from build123d import *

# Parameters (mm, degrees)
SKETCH1_R           = 34.5
BOSS_EXTRUDE1_DEPTH = 3
SKETCH4_R           = 20
CUT_EXTRUDE2_DEPTH  = 49.88251221
SKETCH5_W           = 5
SKETCH5_H           = 5
CUT_EXTRUDE3_DEPTH  = 1.5


with BuildPart() as part:
    # Sketch1 → Boss-Extrude1 (new body)
    with BuildSketch(Plane(origin=(0, 0, 0), x_dir=(1, 0, 0), z_dir=(0, 1, 0))):
        with Locations(Location((0, 0, 0), (0, 0, 270))):
            Circle(SKETCH1_R)
    extrude(amount=BOSS_EXTRUDE1_DEPTH)

    # Sketch4 → Cut-Extrude2 (cut, through all)
    with BuildSketch(Plane(origin=(0, 3, 0), x_dir=(1, 0, 0), z_dir=(0, 1, 0))):
        with Locations(Location((0, 0, 0), (0, 0, 270))):
            Circle(SKETCH4_R)
    extrude(amount=-CUT_EXTRUDE2_DEPTH, mode=Mode.SUBTRACT)

    # Sketch5 → Cut-Extrude3 (cut)
    with BuildSketch(Plane(origin=(0, 3, 0), x_dir=(1, 0, 0), z_dir=(0, 1, 0))):
        with Locations((19.603168608, 19.636741271)):
            Rectangle(SKETCH5_W, SKETCH5_H)
        with Locations((-19.636741271, 19.603168608)):
            Rectangle(SKETCH5_W, SKETCH5_H)
        with Locations((19.636741271, -19.603168608)):
            Rectangle(SKETCH5_W, SKETCH5_H)
        with Locations((-19.603168608, -19.636741271)):
            Rectangle(SKETCH5_W, SKETCH5_H)
    extrude(amount=-CUT_EXTRUDE3_DEPTH, mode=Mode.SUBTRACT)


solid = part.part
Geometry check sheet. Reference: the model listing, model coordinates, mm. A direction names the side the tool comes from. Round coordinates to 2 decimals unless told otherwise and drop trailing zeros. Loops run counter-clockwise (first coordinate to the right, second up) from the corner with the lowest first, then second, coordinate; pieces in that order, holes last.
Item 1: Cross-section at A-A on z = 0. Record the boundary of the cut face in (x, y).
Item 2: Cross-section at C-C on y = 2.55. Record the boundary of the cut face in (x, z), then the cut area to 3 significant figures.
Item 3: Mould release check, pull along X, two halves, no side actions. Record for faces 3 (the flat face through (-15, 3, 15)), 4 (the flat face through (20, 2, 22.103)), 5 (the cylindrical face through (1.517, 1.479, -34.467)): pulls with the +X half, pulls with the -X half, needs draft (parallel to the pull), parting line crosses it, or undercut.
Item 4: Cross-section at B-B on x = 0. Record the boundary of the cut face in (y, z), then the cut area to 3 significant figures.
Item 5: Cross-section at D-D on x = 18. Record the boundary of the cut face in (y, z), then the cut area to 3 significant figures.
Item 6: Thickness scan on line 1 (X direction, y = 2.2, z = 0); line 2 (X direction, y = 0.5, z = 9); line 3 (Z direction, x = -4.5, y = 0.6). Record the ranges inside material, lowest first.
Item 7: Access from +Z, -Z, +X, -X, +Y, -Y to the whole of each face (thin tool, end or side, straight path). Record for faces 1 (the flat face through (-20, 1.5, -20)), 2 (the cylindrical face through (-19.524, 1.521, -4.336)).
Item 8: Gauge pin test, flat ends, axial feed: pin 1 (0.8 mm diameter, centred on x = -21, y = 2, fed in from +Z); pin 2 (1.2 mm diameter, centred on x = -20.5, y = 2.5, fed in from +Z); pin 3 (1.6 mm diameter, centred on x = -18.5, y = 2.5, fed in from -Z). Record the tip position at first contact, or that the pin passes through.
Answer sheet:
1. outline: (-34.5, 0) - (-20, 0) - (-20, 3) - (-34.5, 3) - close; (20, 0) - (34.5, 0) - (34.5, 3) - (20, 3) - close
2. outline: circle Ø69 at (0, 0); hole (-22.14, -22.1) - (-17.14, -22.1) - (-17.14, -17.1) - (-22.14, -17.1) - close; hole (-22.1, 17.14) - (-17.1, 17.14) - (-17.1, 22.14) - (-22.1, 22.14) - close; hole circle Ø40 at (0, 0); hole (17.1, -22.14) - (22.1, -22.14) - (22.1, -17.14) - (17.1, -17.14) - close; hole (17.14, 17.1) - (22.14, 17.1) - (22.14, 22.1) - (17.14, 22.1) - close
2. area: 2,380 mm2
3. face 3: needs draft
3. face 4: undercut
3. face 5: parting line crosses it
4. outline: (0, -34.5) - (3, -34.5) - (3, -20) - (0, -20) - close; (0, 20) - (3, 20) - (3, 34.5) - (0, 34.5) - close
4. area: 87.0 mm2
5. outline: (0, -29.43) - (3, -29.43) - (3, -22.14) - (1.5, -22.14) - (1.5, -17.14) - (3, -17.14) - (3, -8.72) - (0, -8.72) - close; (0, 8.72) - (3, 8.72) - (3, 17.1) - (1.5, 17.1) - (1.5, 22.1) - (3, 22.1) - (3, 29.43) - (0, 29.43) - close
5. area: 109 mm2
6. line 1: x = -34.5 to -20, 20 to 34.5
6. line 2: x = -33.31 to -17.86, 17.86 to 33.31
6. line 3: z = -34.21 to -19.49, 19.49 to 34.21
7. face 1: +Y
7. face 2: +Y, -Y
8. pin 1: stops at z = 27.67
8. pin 2: stops at z = 28.18
8. pin 3: stops at z = -29.61
